Geometry: final body of the model. Coordinates: model frame, mm. A direction names the side the tool comes from. Coordinates: 2 decimals unless noted, no trailing zeros. Write each loop counter-clockwise with the first axis right and the second up, starting at its lowest first coordinate (ties: lowest second). Pieces come first, ordered by that corner, then holes. Notation, with made-up numbers: (73, 72) - (83, 72) arc R16 ccw to (83, 98) - close; hole circle Ø11 at (4, 55). An arc over 180 degrees is marked (long way). Put each result on its own line as item: value.
```python
from build123d import *

# Parameters (mm, degrees)
F0_R      = 6.35
F1_DEPTH  = 25.4
F1_FACE_R = 6.35
F2_DEPTH  = 13.97


with BuildPart() as f1:
    # F0 (on Front) → F1 (new body)
    with BuildSketch(Plane.XZ):
        with BuildLine():
            ThreePointArc((29.115278, -12.663454), (31.084342, -6.467318), (31.75, 0))
            ThreePointArc((31.75, 0), (30.930583, 7.166695), (28.514629, 13.963467))
            ThreePointArc((28.514629, 13.963467), (-31.741925, -0.716033), (29.115278, -12.663454))
        make_face()
        Circle(F0_R, mode=Mode.SUBTRACT)
        with BuildLine():
            ThreePointArc((28.514629, 13.963467), (30.930583, 7.166695), (31.75, 0))
            ThreePointArc((31.75, 0), (31.084342, -6.467318), (29.115278, -12.663454))
            Line((29.115278, -12.663454), (89.507588, -12.663454))
            Line((89.507588, -12.663454), (89.507588, 13.963467))
            Line((89.507588, 13.963467), (28.514629, 13.963467))
        make_face()
    extrude(amount=F1_DEPTH)

    # F1_face (on face) → F2 (join)
    with BuildSketch(Plane(origin=(20.425137, -25.4, 0.228165), x_dir=(1, 0, 0), z_dir=(0, -1, 0))):
        with BuildLine():
            ThreePointArc((8.089492, 13.735302), (-52.167062, -0.944198), (8.690141, -12.891619))
            Line((8.690141, -12.891619), (69.082451, -12.891619))
            Line((69.082451, -12.891619), (69.082451, 13.735302))
            Line((69.082451, 13.735302), (8.089492, 13.735302))
        make_face()
        with Locations((-20.425137, -0.228165)):
            Circle(F1_FACE_R, mode=Mode.SUBTRACT)
    extrude(amount=-F2_DEPTH)


solid = f1.part
```
1. Pin query (flat end, axial travel): pin 1 Ø12 at (y, z) = (-12, 20.5) entering from +X; pin 2 Ø10 at (x, z) = (32.5, 10) entering from +Y; pin 3 Ø7.5 at (x, y) = (60.5, -10) entering from +Z; pin 4 Ø6 at (y, z) = (-14, -23) entering from -X. Return the tip coordinate at first contact, or that it passes through.
Answer below:
pin 1: stops at x = 28.25
pin 2: stops at y = 0
pin 3: stops at z = 13.96
pin 4: stops at x = -24.66
2. Section query D-D (x = 37). Return loops of the section in (y, z), then the cut area to 3 significant figures.
Answer below:
outline: (-25.4, -12.66) - (0, -12.66) - (0, 13.96) - (-25.4, 13.96) - close
area: 676 mm²
3. Section query C-C (y = -7.25). Return loops of the section in (x, z).
Answer below:
outline: (28.51, 13.96) arc R31.75 ccw (long way) to (29.12, -12.66) - (89.51, -12.66) - (89.51, 13.96) - close; hole circle Ø12.7 at (0, 0)
4. Section query B-B (z = 0). Return loops of the section in (x, y).
Answer below:
outline: (-31.75, -25.4) - (-6.35, -25.4) - (-6.35, 0) - (-31.75, 0) - close; (6.35, -25.4) - (89.51, -25.4) - (89.51, 0) - (6.35, 0) - close
5. Set-up query: faces 1 (the cylindrical face through (-31.746, -12.522, 0.488)), 2 (the flat face through (59, -13, -12.663)). Return all of +Z, -Z, +X, -X, +Y, -Y with unobstructed straight access to the full face (end or side cutting, diameter ignored); none if empty.
Answer below:
face 1: +Y, -Y
face 2: -Z, +X, +Y, -Y
6. Section query A-A (x = 0). Return loops of the section in (y, z).
Answer below:
outline: (-25.4, -31.75) - (0, -31.75) - (0, -6.35) - (-25.4, -6.35) - close; (-25.4, 6.35) - (0, 6.35) - (0, 31.75) - (-25.4, 31.75) - close
7. Mould query, pull axis Z, two halves, no side actions, for faces 3 (the flat face through (15, -25.4, 0)), 4 (the flat face through (59, -13, 13.963)), 5 (the cylindrical face through (-1.38, -12.52, -6.2)). Classes: +Z half, -Z half, draft (parallel to the pull), parting line (faces both ways), or undercut.
Answer below:
face 3: draft
face 4: +Z half
face 5: undercut
8. Ray query, probe 1 along Z at (x, y) = (0, -8.75); probe 2 along Z at (x, y) = (76.5, -1.5); probe 3 along Z at (x, y) = (-2, -6.5). Return the intervals inside material, ascending. Write a range as from..to.
Answer below:
probe 1: z = -31.75..-6.35, 6.35..31.75
probe 2: z = -12.66..13.96
probe 3: z = -31.69..-6.03, 6.03..31.69
